from build123d import *

# Parameters (mm, degrees)
SKETCH_1_R          = 1.55
EXTRUDE_1_DEPTH     = 2
CUT_EXTRUDE_2_DEPTH = 33.018928501
EXTRUDE_START       = -2
EXTRUDE_3_DEPTH     = 2
FILLET_1_R          = 3
FILLET_2_R          = 1
SKETCH_5_R          = 0.75
CUT_EXTRUDE_3_DEPTH = 10


with BuildPart() as part:
    # 草图1 → 凸台-拉伸1 (new body)
    with BuildSketch(Plane(origin=(0, 0, 0), x_dir=(1, 0, 0), z_dir=(0, 1, 0))):
        with BuildLine():
            Line((-9.427629845, 12.118007633), (-14.205972572, 5.57250637))
            ThreePointArc((-14.205972572, 5.57250637), (-13.333741258, -0.01669863), (-7.744536258, 0.855532684))
            Line((-7.744536258, 0.855532684), (-2.966193531, 7.401033946))
            ThreePointArc((-2.966193531, 7.401033946), (2.156455687, 5.844533995), (7.508476858, 5.702771934))
            Line((7.508476858, 5.702771934), (9.973957748, -2.017173013))
            ThreePointArc((9.973957748, -2.017173013), (15.001264118, -4.610663069), (17.594754173, 0.416643301))
            Line((17.594754173, 0.416643301), (15.129273283, 8.136588247))
            Line((15.129273283, 8.136588247), (19.53886034, 20.548398832))
            ThreePointArc((19.53886034, 20.548398832), (2.94865648, 10.730730666), (-9.689752685, 25.287244194))
            Line((-9.689752685, 25.287244194), (-9.427629845, 12.118007633))
        make_face()
        with Locations(Location((13.784355961, -0.800264856, 0), (0, 0, 270))):
            Circle(SKETCH_1_R, mode=Mode.SUBTRACT)
        with Locations(Location((-10.975254415, 3.214019527, 0), (0, 0, 270))):
            Circle(SKETCH_1_R, mode=Mode.SUBTRACT)
    extrude(amount=EXTRUDE_1_DEPTH)

    # 草图4 → 切除-拉伸2 (cut, through all)
    with BuildSketch(Plane(origin=(0, 2, 0), x_dir=(1, 0, 0), z_dir=(0, 1, 0))):
        with BuildLine():
            Line((-9.427629845, 12.118007633), (-7.676415353, 18.061742765))
            ThreePointArc((-7.676415353, 18.061742765), (-9.140437111, 21.54705512), (-9.689752685, 25.287244194))
            Line((-9.689752685, 25.287244194), (-9.427629845, 12.118007633))
        make_face()
        with BuildLine():
            ThreePointArc((19.53886034, 20.548398832), (19.021588119, 19.278904179), (18.3909493, 18.061742765))
            Line((18.3909493, 18.061742765), (15.129273283, 8.136588247))
            Line((15.129273283, 8.136588247), (19.53886034, 20.548398832))
        make_face()
    extrude(amount=-CUT_EXTRUDE_2_DEPTH, mode=Mode.SUBTRACT)

    # 草图4<3> → 凸台-拉伸3 (add)
    with BuildSketch(Plane(origin=(0, 2, 0), x_dir=(1, 0, 0), z_dir=(0, 1, 0)).offset(EXTRUDE_START)):
        with BuildLine():
            ThreePointArc((-7.676415353, 18.061742765), (-2.167733027, 12.553060438), (5.357266973, 10.536742765))
            Line((5.357266973, 10.536742765), (-7.676415353, 18.061742765))
        make_face()
        with BuildLine():
            ThreePointArc((5.357266973, 10.536742765), (12.882266973, 12.553060438), (18.3909493, 18.061742765))
            Line((18.3909493, 18.061742765), (5.357266973, 10.536742765))
        make_face()
    extrude(amount=EXTRUDE_3_DEPTH)

    # 圆角1
    fillet_1_edges = [part.edges().sort_by_distance(p)[0] for p in [
        (-9.427629845, 1, -12.118007633),
        (15.129273283, 1, -8.136588247),
        (7.508476858, 1, -5.702771934),
        (-2.966193531, 1, -7.401033946),
    ]]
    fillet(fillet_1_edges, radius=FILLET_1_R)

    # 圆角2
    fillet_2_edges = [part.edges().sort_by_distance(p)[0] for p in [
        (-7.676415353, 1, -18.061742765),
        (18.3909493, 1, -18.061742765),
    ]]
    fillet(fillet_2_edges, radius=FILLET_2_R)

    # 草图5 → 切除-拉伸3 (cut)
    with BuildSketch(Plane(origin=(0, 2, 0), x_dir=(1, 0, 0), z_dir=(0, 1, 0))):
        with Locations(Location((12.263220764, 3.962732909, 0), (0, 0, 270))):
            Circle(SKETCH_5_R)
    extrude(amount=-CUT_EXTRUDE_3_DEPTH, mode=Mode.SUBTRACT)


solid = part.part
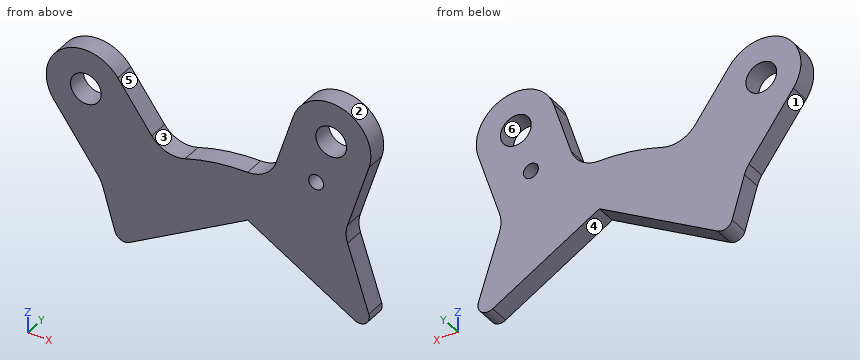
Input: part model. Units: mm. Frame: model coordinates. Face numbers are marked on the shaded views. A direction names the side the tool comes from. Round coordinates to 2 decimals unless told otherwise and drop trailing zeros. Order: outer loops, then holes, each group sorted by start corner. A loop starts at its lowest first (then second) coordinate and runs counter-clockwise, first axis right, second up.
1. Mould query, pull axis X, two halves, no side actions, for the marked faces 1, 2 and 3. Classes: released by +X, released by -X, zero draft, split by the parting line, or undercut.
The answers:
face 1: released by -X
face 2: split by the parting line
face 3: undercut
2. Cut plane B-B, the plane z = -8. Output: boundary loops of the cut face in (x, y).
The answers:
outline: (-12.43, 0) - (15.29, 0) - (15.29, 2) - (-12.43, 2) - close
3. Material intervals for line 1 (X direction, y = 0.4, z = 0); line 2 (X direction, y = 1.25, z = -5); line 3 (X direction, y = 1.1, z = -1.25), sorted ascending.
The answers:
line 1: x = -13.36 to -8.59, 9.33 to 12.46, 15.11 to 17.7
line 2: x = -14.55 to -4.72, 7.14 to 16.13
line 3: x = -14.46 to -7.46, 8.93 to 17.33
4. Set-up query: the marked faces 4, 5 and 6. Return all of +Z, -Z, +X, -X, +Y, -Y with unobstructed straight access to the full face (end or side cutting, diameter ignored); none if empty.
The answers:
face 4: -Z, +Y, -Y
face 5: +Z, +Y, -Y
face 6: +Y, -Y
5. Cut plane C-C, the plane x = 9. Output: boundary loops of the cut face in (y, z), then the cut area to 3 significant figures.
The answers:
outline: (0, -12.64) - (2, -12.64) - (2, -1.03) - (0, -1.03) - close
area: 23.2 mm2
6. Cut plane A-A, the plane y = 1.65. Output: boundary loops of the cut face in (x, z).
The answers:
outline: (-14.21, -5.57) - (-9.73, -11.7) arc R3 cw to (-9.28, -12.62) - (-8.04, -16.84) arc R1 ccw to (-6.58, -17.43) - (5.36, -10.54) - (16.12, -16.75) arc R1 ccw to (17.57, -15.57) - (15.43, -9.06) arc R3 cw to (15.42, -7.21) - (17.59, -0.42) arc R4 ccw to (9.97, 2.02) - (8.21, -3.5) arc R3 cw to (5.35, -5.59) arc R20 ccw to (-0.96, -6.61) arc R3 cw to (-4.33, -5.53) - (-7.74, -0.86) arc R4 ccw to start; hole circle Ø3.1 at (-10.98, -3.21); hole circle Ø1.5 at (12.26, -3.96); hole circle Ø3.1 at (13.78, 0.8)
7. Pin query (flat end, axial travel): P1, Ø3, axis at x = 13.78, z = 0.8, coming from the +Y side; P2, Ø1, axis at x = -11, z = -10.5, coming from the -Y side. Return the tip coordinate at first contact, or that it passes through.
The answers:
P1: passes through
P2: stops at y = 0
